```python
from build123d import *

# Parameters (mm, degrees)
F1_DEPTH = 106.68
F2_R     = 20.442047
F3_DEPTH = 151.13


with BuildPart() as f1:
    # F0 (on Top) → F1 (new body)
    with BuildSketch(Plane.XY):
        with BuildLine():
            Line((0, 0), (28.845539, 0))
            ThreePointArc((28.845539, 0), (26.490793, 11.415035), (19.811004, 20.966383))
            Line((19.811004, 20.966383), (0, 0))
        make_face()
        with BuildLine():
            ThreePointArc((20.966383, -19.811004), (26.803468, -10.660171), (28.845539, 0))
            Line((28.845539, 0), (0, 0))
            Line((0, 0), (20.966383, -19.811004))
        make_face()
        with BuildLine():
            Line((0, 0), (19.811004, 20.966383))
            ThreePointArc((19.811004, 20.966383), (10.660171, 26.803468), (0, 28.845539))
            Line((0, 28.845539), (0, 0))
        make_face()
        with BuildLine():
            ThreePointArc((0, -28.845539), (11.415035, -26.490793), (20.966383, -19.811004))
            Line((20.966383, -19.811004), (0, 0))
            Line((0, 0), (0, -28.845539))
        make_face()
        with BuildLine():
            Line((-19.811004, -20.966383), (0, 0))
            Line((0, 0), (-28.845539, 0))
            ThreePointArc((-28.845539, 0), (-26.490793, -11.415035), (-19.811004, -20.966383))
        make_face()
        with BuildLine():
            Line((-20.966383, 19.811004), (0, 0))
            Line((0, 0), (0, 28.845539))
            ThreePointArc((0, 28.845539), (-11.415035, 26.490793), (-20.966383, 19.811004))
        make_face()
        with BuildLine():
            Line((-28.845539, 0), (0, 0))
            Line((0, 0), (-20.966383, 19.811004))
            ThreePointArc((-20.966383, 19.811004), (-26.803468, 10.660171), (-28.845539, 0))
        make_face()
        with BuildLine():
            Line((0, -28.845539), (0, 0))
            Line((0, 0), (-19.811004, -20.966383))
            ThreePointArc((-19.811004, -20.966383), (-10.660171, -26.803468), (0, -28.845539))
        make_face()
    extrude(amount=F1_DEPTH)

    # F2 (on face) → F3 (cut)
    with BuildSketch(Plane.XY.offset(106.68)):
        Circle(F2_R)
    extrude(amount=-F3_DEPTH, mode=Mode.SUBTRACT)


solid = f1.part
```
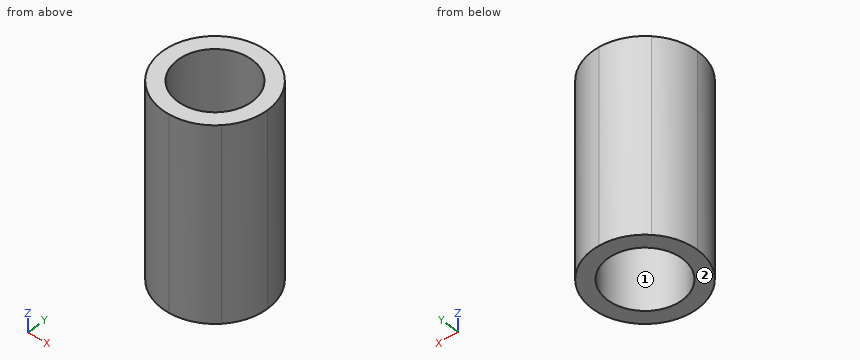
The listing builds one solid part. Answer for the finished solid, in the listing's coordinates (mm). Face numbers are marked on the shaded views. Coordinates: 2 decimals unless noted, no trailing zeros. Loops run counter-clockwise (first coordinate to the right, second up) from the corner with the lowest first, then second, coordinate; pieces in that order, holes last. Notation, with made-up numbers: M 36.25,34 L 40.25,34 A17 ccw 40.25,54 Z; hole C 2.5,38 d1. An arc over 180 degrees is marked long. Answer as a JSON object with one key per item and string values. Group by question number.
Item 1: Section D-D (y = 25) is taken. Write down the section's boundary in (x, z).
Item 2: Section A-A (x = -9) is taken. Write down the section's boundary in (y, z).
Item 3: Section B-B (z = 97.5) is taken. Write down the section's boundary in (x, y), and give its area (3 significant figures).
Item 4: Consider L1, parallel to Y at x = 0, z = 78.5; L2, parallel to X at y = -1, z = 85.5; L3, parallel to X at y = 18, z = 18. Determine where each line is inside the solid, lowest interval first.
Item 5: Section C-C (y = 18.5) is taken. Write down the section's boundary in (x, z).
Item 6: Each of these flat-tipped pins is pushed along its axis until it touches: P1, Ø8, axis at y = -2, z = 78, coming from the +X side; P2, Ø6, axis at x = -14, z = 71.5, coming from the -Y side; P3, Ø2, axis at y = -3.5, z = 41, coming from the +X side; P4, Ø10, axis at x = -13, z = 66, coming from the -Y side. Where does it stop, or does it pass through?
Item 7: Determine the mould class of the marked faces 1 and 2 for opening direction X: +X half, -X half, draft (parallel to the pull), parting line (faces both ways), or undercut.
Solved:
{
 "1": {"outline": "M -14.39,0 L 14.39,0 L 14.39,106.68 L -14.39,106.68 Z"},
 "2": {"outline": "M -27.41,0 L -18.35,0 L -18.35,106.68 L -27.41,106.68 Z; M 18.35,0 L 27.41,0 L 27.41,106.68 L 18.35,106.68 Z"},
 "3": {"outline": "M -28.85,0 A28.85 ccw -19.81,-20.97 A28.85 ccw 0,-28.85 A28.85 ccw 20.97,-19.81 A28.85 ccw 28.85,0 A28.85 ccw 19.81,20.97 A28.85 ccw 0,28.85 A28.85 ccw -20.97,19.81 A28.85 ccw Z; hole C 0,0 d40.88", "area": "1,300 mm2"},
 "4": {"L1": "y = -28.85 to -20.44, 20.44 to 28.85", "L2": "x = -28.83 to -20.42, 20.42 to 28.83", "L3": "x = -22.54 to -9.69, 9.69 to 22.54"},
 "5": {"outline": "M -22.13,0 L -8.7,0 L -8.7,106.68 L -22.13,106.68 Z; M 8.7,0 L 22.13,0 L 22.13,106.68 L 8.7,106.68 Z"},
 "6": {"P1": "stops at x = 28.85", "P2": "stops at y = -26.67", "P3": "stops at x = 28.74", "P4": "stops at y = -27.71"},
 "7": {"face 1": "undercut", "face 2": "draft"}
}
